Work out the finished part from the listing and answer in its coordinate system (mm). Face numbers are marked on the shaded views. A direction names the side the tool comes from. Give positions to 0.01 mm unless a question says otherwise; leave off trailing zeros. Loops run counter-clockwise (first coordinate to the right, second up) from the corner with the lowest first, then second, coordinate; pieces in that order, holes last. Notation, with made-up numbers: M -15.5,4 L -0.5,4 A24 cw -0.5,26 Z; hole C -15,86.25 d10. An arc over 180 degrees is marked long. Answer in a Markdown table with one row per item. Add a question column.
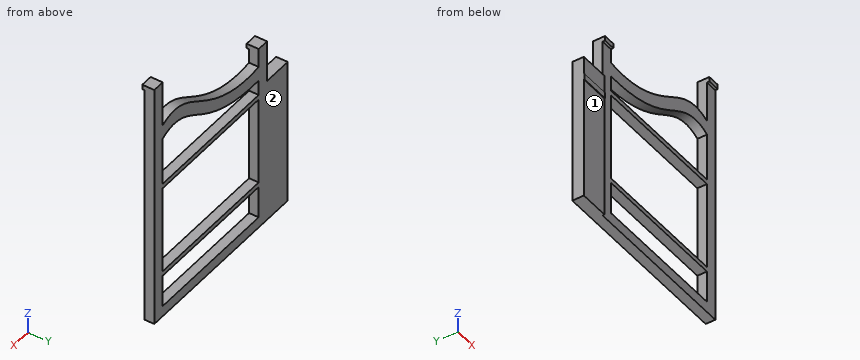
from build123d import *

# Parameters (mm, degrees)
F0_W     = 73.152
F0_H     = 5.744279672
F1_DEPTH = 5.08
F0_W_2   = 6.35
F0_H_2   = 2.54
F0_W_3   = 15.748
F0_H_3   = 3.1443536282
F2_DEPTH = 6.35
F0_H_4   = 9.6294713412
F0_H_5   = 65.5344708799
F3_DEPTH = 6.096
F4_DEPTH = 5.08
F5_DEPTH = 5.08


with BuildPart() as f1:
    # F0 (on Front) → F1 (new body)
    with BuildSketch(Plane.XZ):
        with BuildLine():
            add(Edge.make_bspline(
                [(-61.3806553816, 58.3893715901), (-43.8441733015, 55.5345989136), (-19.0644229117, 66.1410851266), (0, 81.7292685512), (11.7713446184, 75.597518316)],
                knots=[0, 0, 0, 0, 0.5425588266, 1, 1, 1, 1], degree=3))
            Line((-61.3806553816, 58.3893715901), (-61.3806553816, 50.7693715901))
            add(Edge.make_bspline(
                [(-61.3806553816, 50.7693715901), (-44.0213347189, 49.9104853444), (-20.1279301639, 57.0149364757), (0.0923789407, 74.6247452568), (11.7713446184, 67.977518316)],
                knots=[0, 0, 0, 0, 0.5368571136, 1, 1, 1, 1], degree=3))
            Line((11.7713446184, 67.977518316), (11.7713446184, 75.597518316))
        make_face()
        Polygon((-67.7306553816, 65.9703469514), (-67.7306553816, 46.1095218752), (-67.7306553816, 36.480050534), (-67.7306553816, 33.3356969059), (-67.7306553816, -32.198773974), (-61.3806553816, -32.198773974), (-61.3806553816, -26.454494302), (-61.3806553816, -9.338773974), (-61.3806553816, -6.798773974), (-61.3806553816, -1.905), (-61.3806553816, -0.9525), (-61.3806553816, 0), (-61.3806553816, 10.16), (-61.3806553816, 11.1125), (-61.3806553816, 12.065), (-61.3806553816, 40.037518316), (-61.3806553816, 42.577518316), (-61.3806553816, 43.1493715901), (-61.3806553816, 50.7693715901), (-61.3806553816, 58.3893715901), (-61.3806553816, 65.9703469514), align=None)
        with Locations((-24.8046553816, -29.326634138)):
            Rectangle(F0_W, F0_H)
        Polygon((11.7713446184, 97.341226026), (11.7713446184, 75.597518316), (11.7713446184, 67.977518316), (11.7713446184, 46.1095218752), (11.7713446184, 42.577518316), (11.7713446184, 40.037518316), (11.7713446184, 12.065), (11.7713446184, 11.1125), (11.7713446184, 10.16), (11.7713446184, 0), (11.7713446184, -0.9525), (11.7713446184, -1.905), (11.7713446184, -6.798773974), (11.7713446184, -9.338773974), (11.7713446184, -26.454494302), (11.7713446184, -32.198773974), (18.1213446184, -32.198773974), (18.1213446184, 97.341226026), align=None)
    extrude(amount=F1_DEPTH)

    # F0 (on Front) → F2 (join)
    with BuildSketch(Plane.XZ):
        with Locations((-64.5556553816, 67.2403469514)):
            Rectangle(F0_W_2, F0_H_2)
        with Locations((14.9463446184, 98.611226026)):
            Rectangle(F0_W_2, F0_H_2)
        with Locations((-75.6046553816, 34.9078737199)):
            Rectangle(F0_W_3, F0_H_3)
    extrude(amount=F2_DEPTH)

    # F0 (on Front) → F3 (join)
    with BuildSketch(Plane.XZ):
        with Locations((-75.6046553816, 41.2947862046)):
            Rectangle(F0_W_3, F0_H_4)
        with Locations((-75.6046553816, 0.5684614659)):
            Rectangle(F0_W_3, F0_H_5)
    extrude(amount=F3_DEPTH)

    # F0 (on Front) → F4 (join)
    with BuildSketch(Plane.XZ):
        with Locations((-24.8046553816, 41.307518316)):
            Rectangle(F0_W, F0_H_2)
    extrude(amount=F4_DEPTH)

    # F0 (on Front) → F5 (join)
    with BuildSketch(Plane.XZ):
        with Locations((-24.8046553816, -8.068773974)):
            Rectangle(F0_W, F0_H_2)
    extrude(amount=F5_DEPTH)


solid = f1.part
(1) Section A-A, the plane z = 17.5 is taken. Determine the outline of the cut face in (x, y).
(2) Section B-B, the plane x = -66 is taken. Determine the outline of the cut face in (y, z), and give its area (3 significant figures).
(3) Which of the six approach directions +Z, -Z, +X, -X, +Y, -Y give full straight-line access (tool end or side, diameter ignored) to the marked faces 1 and 2?
(4) Consider line 1 along X through (y, z) = (-4.5, 35); line 2 along Z through (x, y) = (0.5, -4); line 3 along Z through (x, y) = (-3, -1.25). Determine where each line is inside the solid, lowest interval first. Write a range as from..to.
(5) Section C-C, the plane y = -3.75 is taken. State how many separate pieces and enclosed holes the cut face has, and give its area (3 significant figures).
(6) Each of these flat-tipped pins is pushed along its axis until it touches: P1, Ø2.5, axis at y = -2, z = 49, coming from the -X side; P2, Ø4, axis at x = 5, z = -8.5, coming from the -Y side; P3, Ø1.5, axis at x = -65, z = 52, coming from the +Y side; P4, Ø2.5, axis at x = -37, y = -3, coming from the +Z side. Where does it stop, or does it pass through?
Numbers:
| question | item | result |
|---|---|---|
| 1 | outline | M -83.48,-6.1 L -67.73,-6.1 L -67.73,-5.08 L -61.38,-5.08 L -61.38,0 L -83.48,0 Z; M 11.77,-5.08 L 18.12,-5.08 L 18.12,0 L 11.77,0 Z |
| 2 | outline | M -6.35,65.97 L -5.08,65.97 L -5.08,-32.2 L 0,-32.2 L 0,68.51 L -6.35,68.51 Z |
| 2 | area | 515 mm² |
| 3 | face 1 | -Z, +X, -X, -Y |
| 3 | face 2 | +Z, -Z, +X, -X, +Y |
| 4 | line 1 | x = -83.48..-61.38, 11.77..18.12 |
| 4 | line 2 | z = -32.2..-26.45, -9.34..-6.8, 40.04..42.58, 70.29..77.8 |
| 4 | line 3 | z = -32.2..-26.45, -9.34..-6.8, 40.04..42.58, 69.47..77.02 |
| 5 | separate pieces | 1 |
| 5 | enclosed holes | 3 |
| 5 | area | 4,030 mm² |
| 6 | P1 | stops at x = -67.73 |
| 6 | P2 | stops at y = -5.08 |
| 6 | P3 | stops at y = 0 |
| 6 | P4 | stops at z = 60.31 |
